The listing builds one solid part. Answer for the finished solid, in the listing's coordinates (mm). A direction names the side the tool comes from. Round coordinates to 2 decimals unless told otherwise and drop trailing zeros. Write each loop counter-clockwise with the first axis right and the second up, starting at its lowest first coordinate (ties: lowest second). Pieces come first, ordered by that corner, then holes. Notation, with made-up numbers: (67.5, 58.25) - (83.5, 58.25) arc R17 cw to (83.5, 76.25) - close; hole circle Ø6 at (-1.5, -6.5). An arc over 180 degrees is marked (long way). Return JSON: item names as keys, results as strings. Group by question number.
(1) Determine the mould class of faces 1 (the cylindrical face through (26.46, 35.05, -0.04)), 2 (the flat face through (-7.3, 0.5, 3.175)), 3 (the flat face through (-30.899, 20.292, 0.044)), 4 (the flat face through (31.84, -31.8, 0.04)) for opening direction Y: +Y half, -Y half, draft (parallel to the pull), parting line (faces both ways), or undercut.
(2) Section C-C, the plane y = -26 is taken. Give the number of separate pieces and of enclosed holes in the cut face, then the cut area to 3 significant figures.
(3) Section A-A, the plane y = 0 is taken. Write down the section's boundary in (x, z) (3 decimals).
(4) Find the intervals of material crossed by line 1 along Y through (x, z) = (12.5, 2.25); line 2 along Y through (x, z) = (-23.5, 2); line 3 along Y through (x, z) = (24, 0.75), in increasing order. Write a range as [from, to].
(5) Which of the six approach directions +Z, -Z, +X, -X, +Y, -Y give full straight-line access (tool end or side, diameter ignored) to faces 5 (the flat face through (-30.973, -20.366, 0.044)), 6 (the flat face through (30.899, -20.292, 0.044)), 7 (the flat face through (-20.292, -30.899, 0.044))?
(6) Each of these flat-tipped pins is pushed along its axis until it touches: pin 1 (2.5 mm diameter, centred on x = 10.61, y = -10.61, fed in from +Z); pin 2 (5 mm diameter, centred on x = 10.61, y = 10.61, fed in from +Z); pin 3 (1 mm diameter, centred on y = 17, z = -2, fed in from -X); pin 4 (2 mm diameter, centred on y = 0.5, z = 0.5, fed in from -X). Where does it stop, or does it pass through?
```python
from build123d import *

# Parameters (mm, degrees)
SKETCH1_R                      = 6.5
F_1_4_IN_SHEET_METAL_DEPTH     = 3.175
M4_CLEARANCE_HOLE1_D           = 4.5
M4_CLEARANCE_HOLE1_CSINK_D     = 8
M4_CLEARANCE_HOLE1_CSINK_ANGLE = 90
M5_CLEARANCE_HOLE1_D           = 5.3
F_25_MM_FILLET_R               = 25
F_5_MM_FILLET_R                = 5
F_0_50_MM_CHAMFER_SIZE         = 0.5


with BuildPart() as part:
    # Sketch1 → 1/4 in Sheet Metal (new, symmetric)
    with BuildSketch(Plane.XY):
        Polygon((0, 10.606601718), (26.516504294, 37.123106012), (37.123106012, 26.516504294), (10.606601718, 0), (37.123106012, -26.516504294), (26.516504294, -37.123106012), (0, -10.606601718), (-26.516504294, -37.123106012), (-37.123106012, -26.516504294), (-10.606601718, 0), (-37.123106012, 26.516504294), (-26.516504294, 37.123106012), align=None)
        Circle(SKETCH1_R, mode=Mode.SUBTRACT)
    extrude(amount=F_1_4_IN_SHEET_METAL_DEPTH, both=True)

    # M4 Clearance Hole1 (through all)
    with Locations(Plane.XY.offset(3.175)):
        with Locations((-10.606601718, 10.606601718), (10.606601718, 10.606601718), (10.606601718, -10.606601718), (-10.606601718, -10.606601718)):
            CounterSinkHole(M4_CLEARANCE_HOLE1_D / 2, M4_CLEARANCE_HOLE1_CSINK_D / 2, counter_sink_angle=M4_CLEARANCE_HOLE1_CSINK_ANGLE)

    # M5 Clearance Hole1 (through all)
    with Locations(Plane(origin=(0, 0, -3.175), x_dir=(-1, 0, 0), z_dir=(0, 0, -1))):
        with Locations((-24.748737342, 24.748737342), (24.748737342, 24.748737342), (24.748737342, -24.748737342), (-24.748737342, -24.748737342)):
            Hole(M5_CLEARANCE_HOLE1_D / 2)

    # 25 mm Fillet
    f_25_mm_fillet_edges = [part.edges().sort_by_distance(p)[0] for p in [
        (0, 10.606601718, 0),
        (10.606601718, 0, 0),
        (0, -10.606601718, 0),
        (-10.606601718, 0, 0),
    ]]
    fillet(f_25_mm_fillet_edges, radius=F_25_MM_FILLET_R)

    # 5 mm Fillet
    f_5_mm_fillet_edges = [part.edges().sort_by_distance(p)[0] for p in [
        (26.516504294, 37.123106012, 0),
        (37.123106012, 26.516504294, 0),
        (37.123106012, -26.516504294, 0),
        (26.516504294, -37.123106012, 0),
        (-26.516504294, -37.123106012, 0),
        (-37.123106012, -26.516504294, 0),
        (-37.123106012, 26.516504294, 0),
        (-26.516504294, 37.123106012, 0),
    ]]
    fillet(f_5_mm_fillet_edges, radius=F_5_MM_FILLET_R)

    # 0.50 mm Chamfer
    f_0_50_mm_chamfer_edges = [part.edges().sort_by_distance(p)[0] for p in [
        (-6.5, 0, -3.175),
        (-6.5, 0, 3.175),
        (22.098737342, -24.748737342, -3.175),
        (22.098737342, -24.748737342, 3.175),
        (-27.398737342, -24.748737342, -3.175),
        (-27.398737342, -24.748737342, 3.175),
        (-27.398737342, 24.748737342, -3.175),
        (-27.398737342, 24.748737342, 3.175),
        (22.098737342, 24.748737342, -3.175),
        (22.098737342, 24.748737342, 3.175),
    ]]
    chamfer(f_0_50_mm_chamfer_edges, length=F_0_50_MM_CHAMFER_SIZE)


solid = part.part
```
Working result:
{
 "1": {"face 1": "+Y half", "face 2": "draft", "face 3": "undercut", "face 4": "-Y half"},
 "2": {"separate pieces": "4", "enclosed holes": "0", "area": "193 mm^2"},
 "3": {"outline": "(-20.962, -3.175) - (-7, -3.175) - (-6.5, -2.675) - (-6.5, 2.675) - (-7, 3.175) - (-20.962, 3.175) - close; (6.5, -2.675) - (7, -3.175) - (20.962, -3.175) - (20.962, 3.175) - (7, 3.175) - (6.5, 2.675) - close"},
 "4": {"line 1": "y = [-24.31, -13.03], [-8.18, 8.18], [13.03, 24.31]", "line 2": "y = [-34.04, -27.09], [-22.41, -10.98], [10.98, 22.41], [27.09, 34.04]", "line 3": "y = [-34.37, -27.29], [-22.21, -11.94], [11.94, 22.21], [27.29, 34.37]"},
 "5": {"face 5": "+Z, -Z, -X", "face 6": "+Z, -Z, +X", "face 7": "+Z, -Z, -Y"},
 "6": {"pin 1": "passes through", "pin 2": "stops at z = 1.68", "pin 3": "stops at x = -28.11", "pin 4": "stops at x = -21.01"}
}
